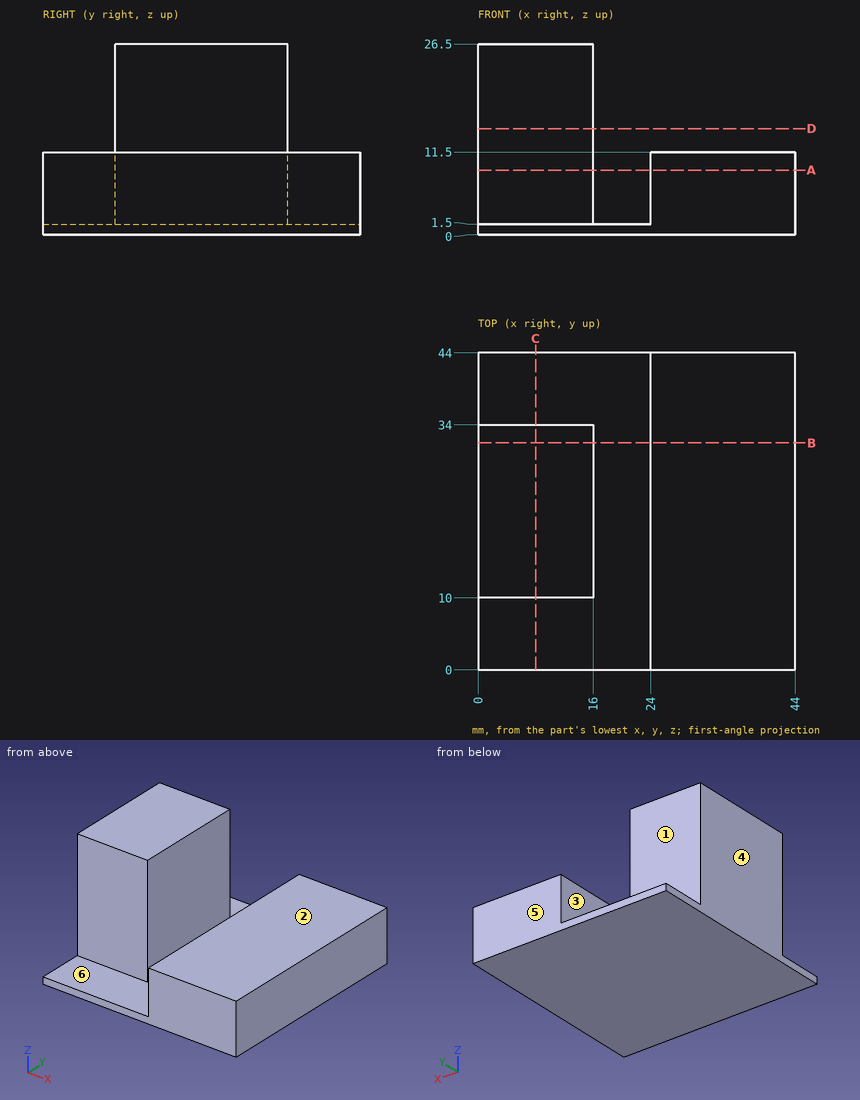
For this review, use the dimensioned drawing (mm, ordinates from the lowest corner) and the shaded views. A direction names the side the tool comes from. Round coordinates to 2 decimals unless told otherwise and drop trailing zeros. Loops run counter-clockwise (first coordinate to the right, second up) from the corner with the lowest first, then second, coordinate; pieces in that order, holes last. Notation, with made-up numbers: M -4,-28.5 L 48,-28.5 A32 cw 48,5.5 Z; hole C 56.5,15.5 d6. An arc over 180 degrees is marked long. Answer as a JSON object with one key per item and string values.
(1) Take a section at A-A on z = 9. Give the boundary of the cut face in (x, y), and give its area (3 significant figures).
Resolved:
{"outline": "M 0,10 L 16,10 L 16,34 L 0,34 Z; M 24,0 L 44,0 L 44,44 L 24,44 Z", "area": "1,260 mm²"}
(2) Draft analysis for pull direction X (two halves, no side actions). For the marked faces 4, 5 and 6, state which applies: released by +X, released by -X, zero draft, split by the parting line, or undercut.
Resolved:
{"face 4": "released by -X", "face 5": "zero draft", "face 6": "undercut"}
(3) Tool access review of the marked faces 1, 2 and 3: name each direction out of +Z, -Z, +X, -X, +Y, -Y from which nothing blocks a thin tool from reaching the whole face with its end or side.
Resolved:
{"face 1": "+Z, -X, +Y", "face 2": "+Z, +X, +Y, -Y", "face 3": "+Z, +Y, -Y"}
(4) Take a section at C-C on x = 8. Give the boundary of the cut face in (y, z), and give its area (3 significant figures).
Resolved:
{"outline": "M 0,0 L 44,0 L 44,1.5 L 34,1.5 L 34,26.5 L 10,26.5 L 10,1.5 L 0,1.5 Z", "area": "666 mm²"}
(5) To check wall thickness, follow line 1 along X through (y, z) = (32.5, 2.25); line 2 along Z through (x, y) = (17, 41); line 3 along Y through (x, z) = (2, 6.25). State the ranges of each line that lie inside material, in increasing order.
Resolved:
{"line 1": "0 to 16, 24 to 44", "line 2": "0 to 1.5", "line 3": "10 to 34"}
(6) Take a section at D-D on z = 14.75. Give the boundary of the cut face in (x, y), and give its area (3 significant figures).
Resolved:
{"outline": "M 0,10 L 16,10 L 16,34 L 0,34 Z", "area": "384 mm²"}
(7) Take a section at B-B on y = 31.5. Give the boundary of the cut face in (x, z), and give its area (3 significant figures).
Resolved:
{"outline": "M 0,0 L 44,0 L 44,11.5 L 24,11.5 L 24,1.5 L 16,1.5 L 16,26.5 L 0,26.5 Z", "area": "666 mm²"}
(8) Clearance check with flat-ended pins moving along their axes: P1, Ø10, axis at x = 17.5, z = 4, coming from the +Y side; P2, Ø10, axis at x = 39.5, y = 32.5, coming from the +Z side; P3, Ø3, axis at y = 20.5, z = 22, coming from the +X side; P4, Ø5, axis at x = 8, z = 17.5, coming from the -Y side. State where each tip first meets the part, or that it passes through.
Resolved:
{"P1": "y = 44", "P2": "z = 11.5", "P3": "x = 16", "P4": "y = 10"}
